Check sheet for the modelled part. Datum: model origin and axes. Units: mm. A direction names the side the tool comes from. Give positions to 0.01 mm unless a question says otherwise; leave off trailing zeros. Write each loop counter-clockwise with the first axis right and the second up, starting at its lowest first coordinate (ties: lowest second). Pieces come first, ordered by that corner, then holes. Notation, with made-up numbers: M -12.75,44 L 7.25,44 A37 ccw 7.25,80 Z; hole C -8,89 d8. An arc over 180 degrees is marked long. Use CSV: the item, a comma, the result in double quotes. Start each with the question number.
1. Mould release check, pull along Y, two halves, no side actions. Record for faces 3 (the face through (57.175, -0.992, -0.044)), 4 (the face through (-68, 6.35, 37)), 5 (the face through (66.675, 0, 0)): +Y half, -Y half, draft (parallel to the pull), parting line (faces both ways), or undercut.
2. Access from +Z, -Z, +X, -X, +Y, -Y to the whole of each face (thin tool, end or side, straight path). Record for faces 1 (the face through (-68, -6.35, 37)), 2 (the face through (-1, 0, 3.175)).
3. Depth check by flat-ended pin: P1, Ø6, axis at x = 60.325, y = 0, coming from the -Z side; P2, Ø6, axis at x = -41, y = 4, coming from the +Z side (3 decimals). Enter the tip coordinate at first touch or a pass-through.
4. Scan lines: line 1 (Z direction, x = -7, y = -1.5) (3 decimals); line 2 (X direction, y = -1.5, z = 84.5) (3 decimals); line 3 (X direction, y = 2.25, z = 58.5) (3 decimals). Record each from-to range of solid material in increasing order.
5. Cross-section at B-B, the plane x = 45. Enter the section's corners in (y, z) (3 decimals).
6. Cross-section at A-A, the plane y = 0. State how many separate pieces and enclosed holes the cut face has, and give its area (3 significant figures).
from build123d import *

# Parameters (mm, degrees)
SKETCH1_W           = 133.35
SKETCH1_H           = 12.7
SKETCH1_R           = 3.302
BOSS_EXTRUDE1_DEPTH = 3.175
BOSS_EXTRUDE2_START = -3.175
SKETCH2_W           = 6.35
SKETCH2_H           = 12.7
BOSS_EXTRUDE2_DEPTH = 127
BOSS_EXTRUDE3_DEPTH = 12.7
LPATTERN1_COUNT     = 50
LPATTERN1_PITCH     = 2.54


with BuildPart() as part:
    # Sketch1 → Boss-Extrude1 (new, symmetric)
    with BuildSketch(Plane.XY):
        Rectangle(SKETCH1_W, SKETCH1_H)
        with Locations((-60.325, 0)):
            Circle(SKETCH1_R, mode=Mode.SUBTRACT)
        with Locations(Location((60.325, 0, 0), (0, 0, 180))):
            Circle(SKETCH1_R, mode=Mode.SUBTRACT)
    extrude(amount=BOSS_EXTRUDE1_DEPTH, both=True)

    # Sketch2 → Boss-Extrude2 (add)
    with BuildSketch(Plane.XY.offset(BOSS_EXTRUDE2_START)):
        with Locations((-69.85, 0)):
            Rectangle(SKETCH2_W, SKETCH2_H)
    extrude(amount=BOSS_EXTRUDE2_DEPTH)

    # Sketch4 → Boss-Extrude3 (add)
    with BuildSketch(Plane(origin=(0, 6.35, 0), x_dir=(1, 0, 0), z_dir=(0, 1, 0))):
        Polygon((-73.025, 3.175), (-75.565, 1.905), (-73.025, 0.635), align=None)
    boss_extrude3 = extrude(amount=-BOSS_EXTRUDE3_DEPTH)

    # LPattern1: Boss-Extrude3 ×50
    with Locations(*[(0, 0, i * LPATTERN1_PITCH) for i in range(1, LPATTERN1_COUNT)]):
        add(boss_extrude3)


solid = part.part
Worked answers:
1,face 3,"undercut"
1,face 4,"+Y half"
1,face 5,"draft"
2,face 1,"+Z, -Z, +X, -X, -Y"
2,face 2,"+Z, +X, +Y, -Y"
3,P1,"passes through"
3,P2,"stops at z = 3.175"
4,line 1,"z = -3.175 to 3.175"
4,line 2,"x = -75.475 to -66.675"
4,line 3,"x = -74.455 to -66.675"
5,outline,"M -6.35,-3.175 L 6.35,-3.175 L 6.35,3.175 L -6.35,3.175 Z"
6,separate pieces,"3"
6,enclosed holes,"0"
6,area,"1,730 mm^2"
